Model file for the job. Use its own axes, mm. Face numbers are marked on the shaded views. A direction names the side the tool comes from. Coordinates: 2 decimals unless noted, no trailing zeros. Loops run counter-clockwise (first coordinate to the right, second up) from the corner with the lowest first, then second, coordinate; pieces in that order, holes last. Notation, with made-up numbers: (-11, 29) -> (23, 29) arc R8 ccw to (23, 43) -> close; hole circle Ø6 at (84, 33.25). An arc over 180 degrees is marked (long way). Use one line per item in the form item = value.
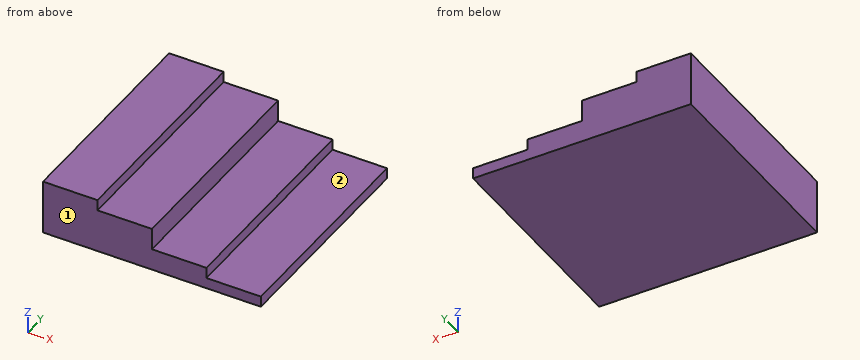
```python
from build123d import *

# Parameters (mm, degrees)
F0_W     = 5
F0_H     = 20
F1_DEPTH = 5
F2_DEPTH = 4
F3_DEPTH = 2
F4_DEPTH = 1


with BuildPart() as f1:
    # F0 (on Top) → F1 (new body)
    with BuildSketch(Plane.XY):
        with Locations((2.5, 10)):
            Rectangle(F0_W, F0_H)
    extrude(amount=F1_DEPTH)

    # F0 (on Top) → F2 (join)
    with BuildSketch(Plane.XY):
        with Locations((7.5, 10)):
            Rectangle(F0_W, F0_H)
    extrude(amount=F2_DEPTH)

    # F0 (on Top) → F3 (join)
    with BuildSketch(Plane.XY):
        with Locations((12.5, 10)):
            Rectangle(F0_W, F0_H)
    extrude(amount=F3_DEPTH)

    # F0 (on Top) → F4 (join)
    with BuildSketch(Plane.XY):
        with Locations((17.5, 10)):
            Rectangle(F0_W, F0_H)
    extrude(amount=F4_DEPTH)


solid = f1.part
```
Q1. Band-saw the part on C-C, the plane z = 3.45. Write the cut outline in (x, y), and give its area (3 significant figures).
Result:
outline = (0, 0) -> (10, 0) -> (10, 20) -> (0, 20) -> close
area = 200 mm2
Q2. Wall check: line 1 along X through (y, z) = (13.75, 2.1); line 2 along Z through (x, y) = (7, 1); line 3 along Z through (x, y) = (14.75, 10.75). Give the ranges that are in metal, low to high.
Result:
line_1 = 0 to 10
line_2 = 0 to 4
line_3 = 0 to 2
Q3. Band-saw the part on B-B, the plane x = 8.25. Write the cut outline in (y, z).
Result:
outline = (0, 0) -> (20, 0) -> (20, 4) -> (0, 4) -> close
Q4. Band-saw the part on A-A, the plane y = 9.25. Write the cut outline in (x, z), and give its area (3 significant figures).
Result:
outline = (0, 0) -> (20, 0) -> (20, 1) -> (15, 1) -> (15, 2) -> (10, 2) -> (10, 4) -> (5, 4) -> (5, 5) -> (0, 5) -> close
area = 60.0 mm2
Q5. Which spindle directions (+Z, -Z, +X, -X, +Y, -Y) get a long thin tool onto all of the face, cutting with end or side? Do the marked faces 1 and 2. Say none if no direction does.
Result:
face_1 = +Z, -Z, +X, -X, -Y
face_2 = +Z, +X, +Y, -Y
Q6. Pin check, flat tips, straight feed: pin 1 Ø2 at (y, z) = (17.5, 2) entering from -X; pin 2 Ø1.5 at (x, y) = (9, 15) entering from +Z; pin 3 Ø1.5 at (x, y) = (13, 11.5) entering from +Z; pin 4 Ø0.8 at (y, z) = (5.5, 4.5) entering from +X. Stop position of each tip, or through.
Result:
pin_1 = 0
pin_2 = 4
pin_3 = 2
pin_4 = 5
